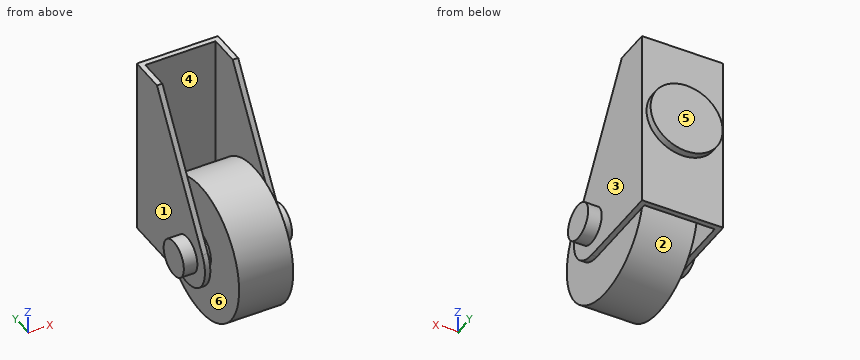
Autodesk Inventor part; units mm, degrees
ref_plane "Work Plane1" through (22.5, 0, 0) normal (1, 0, 0) x (0, 0, -1)
ref_plane "Work Plane2" through (-22.5, 0, 0) normal (-1, 0, 0) x (0, 0, 1)
ref_plane "YZ Plane" through (0, 0, 0) normal (1, 0, 0) x (0, 1, 0)
sketch "Sketch1" plane through (0, 0, 0) normal (1, 0, 0) x (0, 1, 0)
  circle A0 centre (0, 0) radius 38
  dimension "d0" = 76
extrude "Extrusion1" add sketch "Sketch1" along normal mid plane 30
sketch "Sketch2" plane through (0, 0, 0) normal (1, 0, 0) x (0, 1, 0)
  circle A0 centre (0, 0) radius 10
  dimension "d3" = 20
extrude "Extrusion2" add sketch "Sketch2" along normal mid plane 60
ref_plane "Work Plane1" through (22.5, 0, 0) normal (1, 0, 0) x (0, 0, -1)
sketch "Sketch3" plane through (22.5, 0, 0) normal (1, 0, 0) x (0, 0, -1)
  circle A0 centre (0, 0) radius 10
  circle A1 centre (0, 0) radius 10
  circle A2 centre (0, 0) radius 17.5
  line L0 (-82.5, 50) -> (17.5, 50)
  circle A3 centre (0, 0) radius 38
  line L1 (17.5, 0) -> (17.5, 50)
  line L2 (-82.5, 50) -> (-82.5, 30)
  line L3 (-82.5, 30) -> (-9.1391, -14.9241)
  point P0 (-38, 0)
  dimension "d6" = 35
  dimension "d7" = 50
  dimension "d8" = 100
  dimension "d9" = 20
extrude "Extrusion3" add sketch "Sketch3" against normal blind 3 contours A2 | A2 L3 A3 L1 | A3 L3 L2 L0 L1 picked at (-15.7584, 26.6707)
ref_plane "Work Plane2" through (-22.5, 0, 0) normal (-1, 0, 0) x (0, 0, 1)
sketch "Sketch4" plane through (-22.5, 0, 0) normal (-1, 0, 0) x (0, 0, 1)
  line L0 (9.1391, -14.9241) -> (82.5, 30)
  line L1 (82.5, 30) -> (82.5, 50)
  line L2 (82.5, 50) -> (-17.5, 50)
  line L3 (-17.5, 50) -> (-17.5, 0)
  arc A0 (-17.5, 0) -> (9.1391, -14.9241) centre (0, 0) ccw
  circle A1 centre (0, 0) radius 10
extrude "Extrusion4" add sketch "Sketch4" against normal blind 3
sketch "Sketch5" plane through (-22.5, 50, 82.5) normal (0, 1, 0) x (1, 0, 0)
  line L0 (0, 0) -> (0, 100)
  line L1 (0, 0) -> (3, 0)
  line L2 (3, 100) -> (3, 0)
  line L3 (0, 100) -> (3, 100)
  line L4 (45, 100) -> (45, 0)
  line L5 (45, 100) -> (42, 100)
  line L6 (42, 0) -> (42, 100)
  line L7 (45, 0) -> (42, 0)
  line L8 (0, 100) -> (45, 100)
  line L9 (45, 100) -> (45, 0)
  line L10 (45, 0) -> (0, 0)
  line L11 (0, 0) -> (0, 100)
  point P0 (22.5, 82.5)
extrude "Extrusion5" add sketch "Sketch5" against normal blind 3
sketch "Sketch6" plane through (22.5, 50, 82.5) normal (0, 1, 0) x (1, 0, 0)
  line L0 (-37.5, 120.5) -> (-37.5, 44.5)
  line L1 (-7.5, 44.5) -> (-7.5, 120.5)
  line L2 (-37.5, 44.5) -> (-7.5, 44.5) construction
  circle A0 centre (-22.5, 44.5) radius 20
  point P0 (-22.5, 82.5)
  dimension "d16" = 40
extrude "Extrusion6" add sketch "Sketch6" along normal blind 4
properties part number "assist_wheel" material "Steel, Alloy"
Geometry check sheet. Reference: the model listing, model coordinates, mm. Face numbers are marked on the shaded views. A direction names the side the tool comes from. Coordinates: 2 decimals unless noted, no trailing zeros. Order: outer loops, then holes, each group sorted by start corner. A loop starts at its lowest first (then second) coordinate and runs counter-clockwise, first axis right, second up.
Q1. Draft check along X on the marked faces 1, 2 and 3. Enter one of: released by +X, released by -X, zero draft, split by the parting line, or undercut.
Reply:
face 1: released by -X
face 2: undercut
face 3: released by +X
Q2. Sectioned sample at A-A on y = 44. Record the cut outline in (x, z).
Reply:
outline: (-22.5, -17.5) - (-19.5, -17.5) - (-19.5, 82.5) - (-22.5, 82.5) - close; (19.5, -17.5) - (22.5, -17.5) - (22.5, 82.5) - (19.5, 82.5) - close
Q3. Tool access check on the marked faces 4, 5 and 6. Record the directions out of +Z, -Z, +X, -X, +Y, -Y that give a thin tool (end or side, any length) a straight path to the whole face; none if there is none.
Reply:
face 4: +Z, -Z
face 5: +Z, -Z, +X, -X, +Y
face 6: none
Q4. Depth check by flat-ended pin: pin 1 Ø4 at (x, y) = (19, -2.5) entering from +Z; pin 2 Ø1.5 at (x, z) = (-14, -6) entering from +Y; pin 3 Ø12 at (x, y) = (-12.5, 20) entering from +Z. Enter the tip coordinate at first touch or a pass-through.
Reply:
pin 1: stops at z = 32.59
pin 2: stops at y = 50
pin 3: stops at z = 35.33
Q5. Sectioned sample at B-B on z = 0. Record the cut outline in (x, y), and give its area (3 significant figures).
Reply:
outline: (-30, -10) - (-22.5, -10) - (-22.5, -17.5) - (-19.5, -17.5) - (-19.5, -10) - (-15, -10) - (-15, -38) - (15, -38) - (15, -10) - (19.5, -10) - (19.5, -17.5) - (22.5, -17.5) - (22.5, -10) - (30, -10) - (30, 10) - (22.5, 10) - (22.5, 50) - (-22.5, 50) - (-22.5, 10) - (-30, 10) - close; hole (-19.5, 10) - (-15, 10) - (-15, 38) - (15, 38) - (15, 10) - (19.5, 10) - (19.5, 47) - (-19.5, 47) - close
area: 3,280 mm2
Q6. Thickness scan on probe 1 along X at (y, z) = (-14, -5.5); probe 2 along X at (y, z) = (46, 45.5); probe 3 along X at (y, z) = (-19.5, -20.5). Record the ranges inside material, lowest first.
Reply:
probe 1: x = -22.5 to -19.5, -15 to 15, 19.5 to 22.5
probe 2: x = -22.5 to -19.5, 19.5 to 22.5
probe 3: x = -15 to 15
Q7. Sectioned sample at C-C on x = -18. Record the cut outline in (y, z), and give its area (3 significant figures).
Reply:
outline: circle Ø20 at (0, 0); (47, -17.5) - (50, -17.5) - (50, 29.28) - (54, 29.28) - (54, 46.72) - (50, 46.72) - (50, 82.5) - (47, 82.5) - close
area: 684 mm2
Q8. Sectioned sample at D-D on y = 17. Record the cut outline in (x, z).
Reply:
outline: (-22.5, -17.5) - (-19.5, -17.5) - (-19.5, 61.27) - (-22.5, 61.27) - close; (-15, -33.99) - (15, -33.99) - (15, 33.99) - (-15, 33.99) - close; (19.5, -17.5) - (22.5, -17.5) - (22.5, 61.27) - (19.5, 61.27) - close
